Geometry: final body of the model. Coordinates: model frame, mm. A direction names the side the tool comes from. Coordinates: 2 decimals unless noted, no trailing zeros. Write each loop counter-clockwise with the first axis right and the second up, starting at its lowest first coordinate (ties: lowest second). Pieces come first, ordered by that corner, then holes.
from build123d import *

# Parameters (mm, degrees)
F0_W     = 233
F0_H     = 81
F1_DEPTH = 12
F2_W     = 227
F2_H     = 75
F2_R     = 2.4
F2_R_2   = 0.8
F3_DEPTH = 10


with BuildPart() as f1:
    # F0 (on Top) → F1 (new body)
    with BuildSketch(Plane.XY):
        Rectangle(F0_W, F0_H)
    extrude(amount=F1_DEPTH)

    # F2 (on face) → F3 (cut)
    with BuildSketch(Plane.XY.offset(12)):
        Rectangle(F2_W, F2_H)
        with Locations((-95, -19)):
            Circle(F2_R, mode=Mode.SUBTRACT)
        with Locations((95, -19)):
            Circle(F2_R, mode=Mode.SUBTRACT)
        with Locations((-95, 19)):
            Circle(F2_R, mode=Mode.SUBTRACT)
        Circle(F2_R, mode=Mode.SUBTRACT)
        with Locations((95, 19)):
            Circle(F2_R, mode=Mode.SUBTRACT)
        with Locations((-95, 19)):
            Circle(F2_R_2)
        with Locations((-95, -19)):
            Circle(F2_R_2)
        Circle(F2_R_2)
        with Locations((95, 19)):
            Circle(F2_R_2)
        with Locations((95, -19)):
            Circle(F2_R_2)
    extrude(amount=-F3_DEPTH, mode=Mode.SUBTRACT)


solid = f1.part
Item 1: Pin query (flat end, axial travel): pin 1 (0.5 mm diameter, centred on x = -95, y = 19, fed in from +Z). Return the tip coordinate at first contact, or that it passes through.
Derived:
pin 1: stops at z = 2
Item 2: Pull-direction query (X, two-part tool) for faces 3 (the cylindrical face through (-92.783, -19.919, 7.07)), 4 (the flat face through (-2, 37.5, 7)), 5 (the flat face through (-116.5, -1, 6)), 6 (the flat face through (94, -18, 12)); classes: released by +X, released by -X, zero draft, split by the parting line, or undercut.
Derived:
face 3: undercut
face 4: undercut
face 5: released by -X
face 6: zero draft
Item 3: Material intervals for probe 1 along Y at (x, z) = (-95, 9.5); probe 2 along Y at (x, z) = (73.5, 9.25); probe 3 along X at (y, z) = (7, 11.5), sorted ascending.
Derived:
probe 1: y = -40.5 to -37.5, -21.4 to -19.8, -18.2 to -16.6, 16.6 to 18.2, 19.8 to 21.4, 37.5 to 40.5
probe 2: y = -40.5 to -37.5, 37.5 to 40.5
probe 3: x = -116.5 to -113.5, 113.5 to 116.5
Item 4: Section C-C, the plane y = -8.5. Output: boundary loops of the cut face in (x, z), plus the area to 3 significant figures.
Derived:
outline: (-116.5, 0) - (116.5, 0) - (116.5, 12) - (113.5, 12) - (113.5, 2) - (-113.5, 2) - (-113.5, 12) - (-116.5, 12) - close
area: 526 mm2
Item 5: Set-up query: faces 1 (the flat face through (116.5, -1, 6)), 2 (the flat face through (113.5, -1, 7)). Return all of +Z, -Z, +X, -X, +Y, -Y with unobstructed straight access to the full face (end or side cutting, diameter ignored); none if empty.
Derived:
face 1: +Z, -Z, +X, +Y, -Y
face 2: +Z
Item 6: Section A-A, the plane z = 8.25. State how many separate pieces and enclosed holes the cut face has, plus the area to 3 significant figures.
Derived:
separate pieces: 6
enclosed holes: 6
area: 1,930 mm2
Item 7: Section B-B, the plane x = 19.5. Output: boundary loops of the cut face in (y, z).
Derived:
outline: (-40.5, 0) - (40.5, 0) - (40.5, 12) - (37.5, 12) - (37.5, 2) - (-37.5, 2) - (-37.5, 12) - (-40.5, 12) - close
